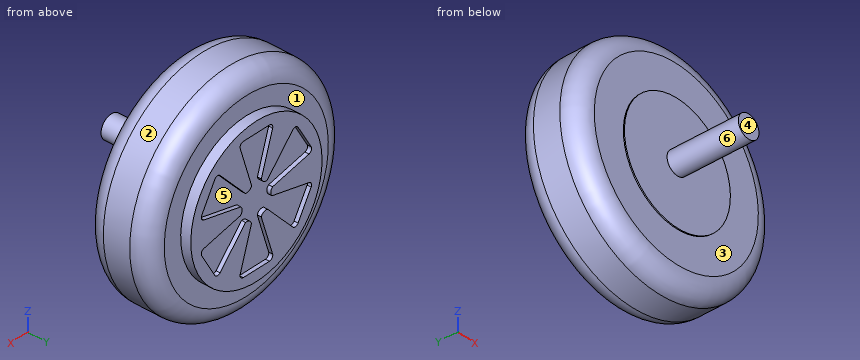
```python
from build123d import *

# Parameters (mm, degrees)
SKETCH3_R           = 76.2
SKETCH3_R_2         = 34.29
BOSS_EXTRUDE1_DEPTH = 43.942
SKETCH4_R           = 41.021
CUT_EXTRUDE1_DEPTH  = 3.556
FILLET1_R           = 12.7
SKETCH5_R           = 50.8
BOSS_EXTRUDE2_DEPTH = 7.112
SKETCH7_R           = 44.45
BOSS_EXTRUDE3_DEPTH = 7.366
CUT_EXTRUDE2_DEPTH  = 2.794
BOSS_EXTRUDE5_DEPTH = 41.91
SKETCH11_R          = 41.021
BOSS_EXTRUDE6_DEPTH = 4.318
SKETCH12_R          = 8
BOSS_EXTRUDE7_DEPTH = 50


with BuildPart() as part:
    # Sketch3 → Boss-Extrude1 (new body)
    with BuildSketch(Plane(origin=(0, 0, 0), x_dir=(1, 0, 0), z_dir=(0, 1, 0))):
        with Locations(Location((0, 0, 0), (0, 0, 90))):
            Circle(SKETCH3_R)
        with Locations(Location((0, 0, 0), (0, 0, 90))):
            Circle(SKETCH3_R_2, mode=Mode.SUBTRACT)
    extrude(amount=BOSS_EXTRUDE1_DEPTH)

    # Sketch4 → Cut-Extrude1 (cut)
    with BuildSketch(Plane(origin=(0, 43.942, 0), x_dir=(1, 0, 0), z_dir=(0, 1, 0))):
        with Locations(Location((0, 0, 0), (0, 0, 270))):
            Circle(SKETCH4_R)
    cut_extrude1 = extrude(amount=-CUT_EXTRUDE1_DEPTH, mode=Mode.SUBTRACT)

    # Mirror1: Cut-Extrude1 across plane
    add(cut_extrude1.mirror(Plane.ZX.offset(21.971)), mode=Mode.SUBTRACT)

    # Fillet1
    fillet1_edges = [part.edges().sort_by_distance(p)[0] for p in [
        (0, 0, 76.2),
        (0, 43.942, 76.2),
    ]]
    fillet(fillet1_edges, radius=FILLET1_R)



with BuildPart() as body_2:
    # Sketch5 → Boss-Extrude2 (new body)
    with BuildSketch(Plane(origin=(0, 43.942, 0), x_dir=(1, 0, 0), z_dir=(0, 1, 0))):
        with Locations(Location((0, 0, 0), (0, 0, 270))):
            Circle(SKETCH5_R)
    extrude(amount=BOSS_EXTRUDE2_DEPTH)

    # Sketch7 → Boss-Extrude3 (add)
    with BuildSketch(Plane(origin=(0, 51.054, 0), x_dir=(1, 0, 0), z_dir=(0, 1, 0))):
        with Locations(Location((0, 0, 0), (0, 0, 270))):
            Circle(SKETCH7_R)
    extrude(amount=-BOSS_EXTRUDE3_DEPTH)

    # Sketch8 → Cut-Extrude2 (cut)
    with BuildSketch(Plane(origin=(0, 51.054, 0), x_dir=(1, 0, 0), z_dir=(0, 1, 0))):
        with BuildLine():
            Line((-3.717986915, 11.786271444), (-12.545239758, 39.769263451))
            ThreePointArc((-12.545239758, 39.769263451), (-12.171377231, 42.035175802), (-10.12290422, 43.073390757))
            Line((-10.12290422, 43.073390757), (10.12290422, 43.073390757))
            ThreePointArc((10.12290422, 43.073390757), (12.171377231, 42.035175802), (12.545239758, 39.769263451))
            Line((12.545239758, 39.769263451), (3.832946747, 12.150701932))
            ThreePointArc((3.832946747, 12.150701932), (5.461454635, 9.696711292), (8.348217029, 9.113006841))
            Line((8.348217029, 9.113006841), (28.16857256, 30.749128053))
            ThreePointArc((28.16857256, 30.749128053), (30.317841482, 31.558309782), (32.241198512, 30.303387593))
            Line((32.241198512, 30.303387593), (42.364102732, 12.770003164))
            ThreePointArc((42.364102732, 12.770003164), (42.489218712, 10.47686602), (40.713812318, 9.020135398))
            Line((40.713812318, 9.020135398), (12.43928992, 2.755921712))
            ThreePointArc((12.43928992, 2.755921712), (11.12832563, 0.11859719), (12.066203944, -2.673264603))
            Line((12.066203944, -2.673264603), (40.713812318, -9.020135398))
            ThreePointArc((40.713812318, -9.020135398), (42.489218712, -10.47686602), (42.364102732, -12.770003164))
            Line((42.364102732, -12.770003164), (32.241198512, -30.303387593))
            ThreePointArc((32.241198512, -30.303387593), (30.317841482, -31.558309782), (28.16857256, -30.749128053))
            Line((28.16857256, -30.749128053), (8.606343173, -9.39478022))
            ThreePointArc((8.606343173, -9.39478022), (5.666870994, -9.578114102), (3.717986915, -11.786271444))
            Line((3.717986915, -11.786271444), (12.545239758, -39.769263451))
            ThreePointArc((12.545239758, -39.769263451), (12.171377231, -42.035175802), (10.12290422, -43.073390757))
            Line((10.12290422, -43.073390757), (-10.12290422, -43.073390757))
            ThreePointArc((-10.12290422, -43.073390757), (-12.171377231, -42.035175802), (-12.545239758, -39.769263451))
            Line((-12.545239758, -39.769263451), (-3.832946747, -12.150701932))
            ThreePointArc((-3.832946747, -12.150701932), (-5.461454635, -9.696711292), (-8.348217029, -9.113006841))
            Line((-8.348217029, -9.113006841), (-28.16857256, -30.749128053))
            ThreePointArc((-28.16857256, -30.749128053), (-30.317841482, -31.558309782), (-32.241198512, -30.303387593))
            Line((-32.241198512, -30.303387593), (-42.364102732, -12.770003164))
            ThreePointArc((-42.364102732, -12.770003164), (-42.489218712, -10.47686602), (-40.713812318, -9.020135398))
            Line((-40.713812318, -9.020135398), (-12.43928992, -2.755921712))
            ThreePointArc((-12.43928992, -2.755921712), (-11.12832563, -0.11859719), (-12.066203944, 2.673264603))
            Line((-12.066203944, 2.673264603), (-40.713812318, 9.020135398))
            ThreePointArc((-40.713812318, 9.020135398), (-42.489218712, 10.47686602), (-42.364102732, 12.770003164))
            Line((-42.364102732, 12.770003164), (-32.241198512, 30.303387593))
            ThreePointArc((-32.241198512, 30.303387593), (-30.317841482, 31.558309782), (-28.16857256, 30.749128053))
            Line((-28.16857256, 30.749128053), (-8.606343173, 9.39478022))
            ThreePointArc((-8.606343173, 9.39478022), (-5.666870994, 9.578114102), (-3.717986915, 11.786271444))
        make_face()
    extrude(amount=-CUT_EXTRUDE2_DEPTH, mode=Mode.SUBTRACT)


with BuildPart() as part_1:
    add(part.part)

    add(body_2.part)  # Boss-Extrude5 merges body 2
    # Sketch10 → Boss-Extrude5 (add)
    with BuildSketch(Plane(origin=(0, 48.26, 0), x_dir=(1, 0, 0), z_dir=(0, 1, 0))):
        with BuildLine():
            Line((10.12290422, 45.613390757), (-10.12290422, 45.613390757))
            ThreePointArc((-10.12290422, 45.613390757), (-14.219850242, 43.536960847), (-14.967575297, 39.005136146))
            Line((-14.967575297, 39.005136146), (-6.471688132, 12.072595881))
            ThreePointArc((-6.471688132, 12.072595881), (-6.854928199, 11.827206148), (-7.29904471, 11.727961017))
            Line((-7.29904471, 11.727961017), (-26.295651132, 32.464868513))
            ThreePointArc((-26.295651132, 32.464868513), (-30.594188976, 34.083231971), (-34.440903038, 31.573387593))
            Line((-34.440903038, 31.573387593), (-44.563807258, 14.040003164))
            ThreePointArc((-44.563807258, 14.040003164), (-44.814039218, 9.453728876), (-41.263226429, 6.540267633))
            Line((-41.263226429, 6.540267633), (-13.691018788, 0.431651613))
            ThreePointArc((-13.691018788, 0.431651613), (-13.67012508, -0.022938888), (-13.80623453, -0.457177633))
            Line((-13.80623453, -0.457177633), (-41.263226429, -6.540267633))
            ThreePointArc((-41.263226429, -6.540267633), (-44.814039218, -9.453728876), (-44.563807258, -14.040003164))
            Line((-44.563807258, -14.040003164), (-34.440903038, -31.573387593))
            ThreePointArc((-34.440903038, -31.573387593), (-30.594188976, -34.083231971), (-26.295651132, -32.464868513))
            Line((-26.295651132, -32.464868513), (-7.219330657, -11.640944268))
            ThreePointArc((-7.219330657, -11.640944268), (-6.81519688, -11.850145036), (-6.507189821, -12.185138651))
            Line((-6.507189821, -12.185138651), (-14.967575297, -39.005136146))
            ThreePointArc((-14.967575297, -39.005136146), (-14.219850242, -43.536960847), (-10.12290422, -45.613390757))
            Line((-10.12290422, -45.613390757), (10.12290422, -45.613390757))
            ThreePointArc((10.12290422, -45.613390757), (14.219850242, -43.536960847), (14.967575297, -39.005136146))
            Line((14.967575297, -39.005136146), (6.471688132, -12.072595881))
            ThreePointArc((6.471688132, -12.072595881), (6.854928199, -11.827206148), (7.29904471, -11.727961017))
            Line((7.29904471, -11.727961017), (26.295651132, -32.464868513))
            ThreePointArc((26.295651132, -32.464868513), (30.594188976, -34.083231971), (34.440903038, -31.573387593))
            Line((34.440903038, -31.573387593), (44.563807258, -14.040003164))
            ThreePointArc((44.563807258, -14.040003164), (44.814039218, -9.453728876), (41.263226429, -6.540267633))
            Line((41.263226429, -6.540267633), (13.691018788, -0.431651613))
            ThreePointArc((13.691018788, -0.431651613), (13.67012508, 0.022938888), (13.80623453, 0.457177633))
            Line((13.80623453, 0.457177633), (41.263226429, 6.540267633))
            ThreePointArc((41.263226429, 6.540267633), (44.814039218, 9.453728876), (44.563807258, 14.040003164))
            Line((44.563807258, 14.040003164), (34.440903038, 31.573387593))
            ThreePointArc((34.440903038, 31.573387593), (30.594188976, 34.083231971), (26.295651132, 32.464868513))
            Line((26.295651132, 32.464868513), (7.219330657, 11.640944268))
            ThreePointArc((7.219330657, 11.640944268), (6.81519688, 11.850145036), (6.507189821, 12.185138651))
            Line((6.507189821, 12.185138651), (14.967575297, 39.005136146))
            ThreePointArc((14.967575297, 39.005136146), (14.219850242, 43.536960847), (10.12290422, 45.613390757))
        make_face()
    extrude(amount=-BOSS_EXTRUDE5_DEPTH)

    # Sketch11 → Boss-Extrude6 (add)
    with BuildSketch(Plane.XZ.offset(-3.556)):
        with Locations(Location((0, 0, 0), (0, 0, 90))):
            Circle(SKETCH11_R)
    extrude(amount=BOSS_EXTRUDE6_DEPTH)

    # Sketch12 → Boss-Extrude7 (add)
    with BuildSketch(Plane.XZ.offset(0.762)):
        with Locations(Location((0, 0, 0), (0, 0, 270))):
            Circle(SKETCH12_R)
    extrude(amount=BOSS_EXTRUDE7_DEPTH)


solid = part_1.part
```
Source: CAD feature listing. Evaluate the final solid. Frame: model axes, mm. Face numbers are marked on the shaded views. A direction names the side the tool comes from. Round coordinates to 2 decimals unless told otherwise and drop trailing zeros. Order: outer loops, then holes, each group sorted by start corner. A loop starts at its lowest first (then second) coordinate and runs counter-clockwise, first axis right, second up. Notation, with made-up numbers: (65.25, 30.5) -> (86.25, 30.5) arc R20 ccw to (86.25, 42.5) -> close; hole circle Ø4 at (70, 27). An arc over 180 degrees is marked (long way). Use CSV: the item, a comma, the result in double quotes.
(1) Section A-A on x = 0. Return the cut outline in (y, z), and give its area (3 significant figures).
Report:
outline,"(-50.76, -8) -> (-0.76, -8) -> (-0.76, -41.02) -> (0, -41.02) -> (0, -63.5) arc R12.7 ccw to (12.7, -76.2) -> (31.24, -76.2) arc R12.7 ccw to (43.94, -63.5) -> (43.94, -50.8) -> (51.05, -50.8) -> (51.05, -43.07) -> (48.26, -43.07) -> (48.26, 43.07) -> (51.05, 43.07) -> (51.05, 50.8) -> (43.94, 50.8) -> (43.94, 63.5) arc R12.7 ccw to (31.24, 76.2) -> (12.7, 76.2) arc R12.7 ccw to (0, 63.5) -> (0, 41.02) -> (-0.76, 41.02) -> (-0.76, 8) -> (-50.76, 8) -> close; hole (3.56, -34.29) -> (6.35, -34.29) -> (6.35, 34.29) -> (3.56, 34.29) -> close"
area,"7,710 mm^2"
(2) Ray query, L1, parallel to X at y = 28, z = 0; L2, parallel to Y at x = -24, z = 5; L3, parallel to Y at x = 2, z = -47.5. Return the intervals inside material, ascending.
Report:
L1,"-76.2 to -34.29, -13.67 to 13.67, 34.29 to 76.2"
L2,"-0.76 to 3.56, 6.35 to 51.05"
L3,"0 to 51.05"
(3) Pull-direction query (X, two-part tool) for the marked faces 4, 5 and 6; classes: +X half, -X half, draft (parallel to the pull), parting line (faces both ways), or undercut.
Report:
face 4,"draft"
face 5,"undercut"
face 6,"parting line"
(4) First-contact query: pin 1 Ø6 at (x, z) = (18, 23.5) entering from -Y; pin 2 Ø3 at (x, y) = (12.5, 29) entering from +Z; pin 3 Ø1 at (y, z) = (40.5, 54) entering from +X. Flat tips, straight axial feed; report the tip coordinate or a pass-through.
Report:
pin 1,"y = -0.76"
pin 2,"z = 75.4"
pin 3,"x = 48.86"
(5) Access query for the marked faces 1, 2 and 3. Directions: +Z, -Z, +X, -X, +Y, -Y. A direction counts if a zero-diameter tool reaches every point of the face in a straight line with its end or side. Return the directions, or none.
Report:
face 1,"+Y"
face 2,"+Y, -Y"
face 3,"-Y"
(6) Section B-B on y = -12.5. Return the cut outline in (x, z).
Report:
outline,"circle Ø16 at (0, 0)"
